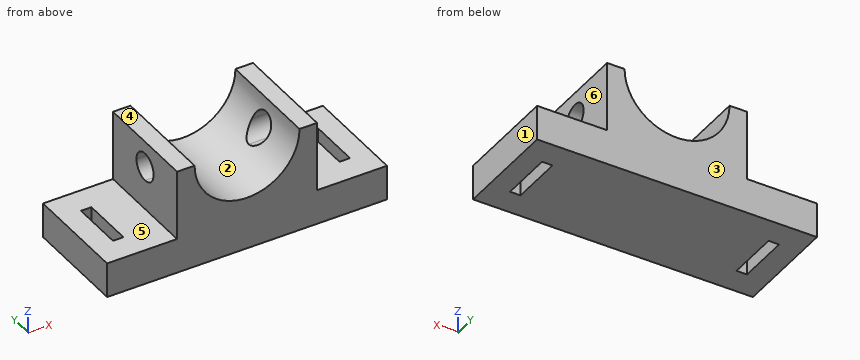
```python
from build123d import *

# Parameters (mm, degrees)
F0_W      = 1600
F0_H      = 600
F1_DEPTH  = 600
F3_DEPTH  = 600.001
F5_W      = 400
F5_H      = 400
F6_DEPTH  = 600.001
F7_W      = 400
F7_H      = 400
F8_DEPTH  = 600.001
F10_DEPTH = 1400
F12_DEPTH = 200.001
F14_DEPTH = 600.001


with BuildPart() as f1:
    # F0 (on Top) → F1 (new body)
    with BuildSketch(Plane.XY):
        Rectangle(F0_W, F0_H)
    extrude(amount=F1_DEPTH)

    # F2 (on face) → F3 (cut, through all)
    with BuildSketch(Plane.XZ.offset(300)):
        with BuildLine():
            ThreePointArc((-300, 600), (0, 300), (300, 600))
            Line((300, 600), (-300, 600))
        make_face()
    extrude(amount=-F3_DEPTH, mode=Mode.SUBTRACT)

    # F5 (on face) → F6 (cut, through all)
    with BuildSketch(Plane.XZ.offset(300)):
        with Locations((600, 400)):
            Rectangle(F5_W, F5_H)
    extrude(amount=-F6_DEPTH, mode=Mode.SUBTRACT)

    # F7 (on face) → F8 (cut, through all)
    with BuildSketch(Plane.XZ.offset(300)):
        with Locations((-600, 400)):
            Rectangle(F7_W, F7_H)
    extrude(amount=-F8_DEPTH, mode=Mode.SUBTRACT)

    # F9 (on face) → F10 (cut)
    with BuildSketch(Plane.YZ.offset(400)):
        with BuildLine():
            ThreePointArc((80, 450), (-56.568542, 506.568542), (0, 370))
            ThreePointArc((0, 370), (56.568542, 393.431458), (80, 450))
        make_face()
    extrude(amount=-F10_DEPTH, mode=Mode.SUBTRACT)

    # F11 (on face) → F12 (cut, through all)
    with BuildSketch(Plane.XY.offset(200)):
        Polygon((680, -150), (680, 0), (680, 150), (620, 150), (620, -150), align=None)
    extrude(amount=-F12_DEPTH, mode=Mode.SUBTRACT)

    # F13 (on face) → F14 (cut, through all)
    with BuildSketch(Plane.XY.offset(600)):
        Polygon((-674.93165, 0), (-674.93165, -150), (-614.93165, -150), (-614.93165, 150), (-674.93165, 150), align=None)
    extrude(amount=-F14_DEPTH, mode=Mode.SUBTRACT)


solid = f1.part
```
Geometry check sheet. Reference: the model listing, model coordinates, mm. Face numbers are marked on the shaded views. A direction names the side the tool comes from. Give positions to 0.01 mm unless a question says otherwise; leave off trailing zeros. Loops run counter-clockwise (first coordinate to the right, second up) from the corner with the lowest first, then second, coordinate; pieces in that order, holes last. Notation, with made-up numbers: (83, -38) - (129, -38) arc R11 ccw to (129, -34) - close; hole circle Ø2 at (39, -4). An arc over 180 degrees is marked (long way). Use CSV: the item, a comma, the result in double quotes. Start each with the question number.
Q1. Scan lines: probe 1 along Y at (x, z) = (-351, 450); probe 2 along Z at (x, y) = (-555, -60); probe 3 along X at (y, z) = (217, 554). Record each from-to range of solid material in increasing order. Write a range as from..to.
Q2. Section check D-D, the plane y = 47.5. Record the cut outline in (x, z).
Q3. Section check A-A, the plane y = -97. Record the cut outline in (x, z).
Q4. Go/stop test with a flat-tipped pin: pin 1 Ø8 at (y, z) = (-134.5, 333.5) entering from +X. Record where the tip stops, or that it passes through.
Q5. Section check B-B, the plane z = 392. Record the cut outline in (x, y), and give its area (3 significant figures).
Q6. Section check C-C, the plane y = 264.5. Record the cut outline in (x, z).
Q7. Release check for a two-part mould opening along X. For the marked faces 1, 2 and 3 record: +X half, -X half, draft (parallel to the pull), parting line (faces both ways), or undercut.
Q8. Access from +Z, -Z, +X, -X, +Y, -Y to the whole of each face (thin tool, end or side, straight path). Record for the marked faces 4, 5 and 6.
Findings below:
1,probe 1,"y = -300..-80, 80..300"
1,probe 2,"z = 0..200"
1,probe 3,"x = -400..-296.45, 296.45..400"
2,outline,"(-800, 0) - (-674.93, 0) - (-674.93, 200) - (-800, 200) - close; (-614.93, 0) - (620, 0) - (620, 200) - (400, 200) - (400, 385.63) - (209.87, 385.63) arc R300 cw to (-209.87, 385.63) - (-400, 385.63) - (-400, 200) - (-614.93, 200) - close; (-400, 514.37) - (-287.52, 514.37) arc R300 cw to (-300, 600) - (-400, 600) - close; (287.52, 514.37) - (400, 514.37) - (400, 600) - (300, 600) arc R300 cw to start; (680, 0) - (800, 0) - (800, 200) - (680, 200) - close"
3,outline,"(-800, 0) - (-674.93, 0) - (-674.93, 200) - (-800, 200) - close; (-614.93, 0) - (620, 0) - (620, 200) - (400, 200) - (400, 600) - (300, 600) arc R300 cw to (-300, 600) - (-400, 600) - (-400, 200) - (-614.93, 200) - close; (680, 0) - (800, 0) - (800, 200) - (680, 200) - close"
4,pin 1,"stops at x = 400"
5,outline,"(-400, -300) - (-216.19, -300) - (-216.19, -55.1) - (-400, -55.1) - close; (-400, 55.1) - (-216.19, 55.1) - (-216.19, 300) - (-400, 300) - close; (216.19, -300) - (400, -300) - (400, -55.1) - (216.19, -55.1) - close; (216.19, 55.1) - (400, 55.1) - (400, 300) - (216.19, 300) - close"
5,area,"180,000 mm^2"
6,outline,"(-800, 0) - (800, 0) - (800, 200) - (400, 200) - (400, 600) - (300, 600) arc R300 cw to (-300, 600) - (-400, 600) - (-400, 200) - (-800, 200) - close"
7,face 1,"+X half"
7,face 2,"undercut"
7,face 3,"draft"
8,face 4,"+Z, +X, -X, +Y, -Y"
8,face 5,"+Z, -X, +Y, -Y"
8,face 6,"+Z, +X, +Y, -Y"
